```python
from build123d import *

# Parameters (mm, degrees)
F2_W     = 4.6
F2_H     = 45
F3_DEPTH = 12.5
F4_W     = 4.6
F4_H     = 45
F5_DEPTH = 12.5


with BuildPart() as f1:
    # F0 (on Right) → F1 (revolve)
    with BuildSketch(Plane.YZ):
        Polygon((-6, 0), (-6, 50), (-8, 50), (-8, 0.018575), (-3.663243, -12), (-2.5, -12), (-2.5, -9.5), align=None)
    revolve(axis=Axis((0, 0, 4.996806), (0, 0, -1)))

    # F2 (on Front) → F3 (cut, symmetric)
    with BuildSketch(Plane.XZ):
        with Locations((0, 22.5)):
            Rectangle(F2_W, F2_H)
    extrude(amount=F3_DEPTH, both=True, mode=Mode.SUBTRACT)

    # F4 (on Right) → F5 (cut, symmetric)
    with BuildSketch(Plane.YZ):
        with Locations((0, 22.5)):
            Rectangle(F4_W, F4_H)
    extrude(amount=F5_DEPTH, both=True, mode=Mode.SUBTRACT)


solid = f1.part
```
Check sheet for the modelled part. Datum: model origin and axes. Units: mm. A direction names the side the tool comes from. Give positions to 0.01 mm unless a question says otherwise; leave off trailing zeros. Loops run counter-clockwise (first coordinate to the right, second up) from the corner with the lowest first, then second, coordinate; pieces in that order, holes last. Notation, with made-up numbers: M 77,45.25 L 136,45.25 A31 cw 136,75.25 Z; hole C 8.5,-11 d3. An arc over 180 degrees is marked long. Answer in a Markdown table with one row per item.
1) Thickness scan on line 1 (X direction, y = -3.5, z = 37.5); line 2 (X direction, y = 0, z = -10.85); line 3 (Y direction, x = -6, z = 39). Record the ranges inside material, lowest first.
Solutions:
| item | result |
|---|---|
| line 1 | x = -7.19 to -4.87, 4.87 to 7.19 |
| line 2 | x = -4.08 to -2.5, 2.5 to 4.08 |
| line 3 | y = -5.29 to -2.3, 2.3 to 5.29 |
2) Cross-section at A-A (z = 12). Enter the section's corners in (x, y), plus the area to 3 significant figures.
Solutions:
| item | result |
|---|---|
| outline | M -7.66,-2.3 A8 ccw -2.3,-7.66 L -2.3,-5.54 A6 cw -5.54,-2.3 Z; M -7.66,2.3 L -5.54,2.3 A6 cw -2.3,5.54 L -2.3,7.66 A8 ccw Z; M 2.3,-7.66 A8 ccw 7.66,-2.3 L 5.54,-2.3 A6 cw 2.3,-5.54 Z; M 2.3,5.54 A6 cw 5.54,2.3 L 7.66,2.3 A8 ccw 2.3,7.66 Z |
| area | 50.5 mm^2 |
3) Cross-section at B-B (x = 0). Enter the section's corners in (y, z).
Solutions:
| item | result |
|---|---|
| outline | M -8,45 L -6,45 L -6,50 L -8,50 Z; M -7.99,0 L -3.66,-12 L -2.5,-12 L -2.5,-9.5 L -6,0 Z; M 2.5,-12 L 3.66,-12 L 7.99,0 L 6,0 L 2.5,-9.5 Z; M 6,45 L 8,45 L 8,50 L 6,50 Z |
4) Depth check by flat-ended pin: pin 1 (1.1 mm diameter, centred on y = 6.5, z = 13, fed in from -X); pin 2 (4 mm diameter, centred on y = -1.5, z = -1.5, fed in from +X); pin 3 (7 mm diameter, centred on x = 0, y = 0, fed in from -Z); pin 4 (0.6 mm diameter, centred on x = -6.5, z = 22, fed in from +Y). Enter the tip coordinate at first touch or a pass-through.
Solutions:
| item | result |
|---|---|
| pin 1 | stops at x = -5.35 |
| pin 2 | stops at x = 7.99 |
| pin 3 | stops at z = -12 |
| pin 4 | stops at y = 5.06 |
5) Tool access check on faces 1 (the face through (-7, 0, 45)), 2 (the face through (-2.3, 7, 22)), 3 (the face through (3.65, 4.76, 25.35)), 4 (the face through (3.06, -7.39, 24.66)). Record the directions out of +Z, -Z, +X, -X, +Y, -Y that give a thin tool (end or side, any length) a straight path to the whole face; none if there is none.
Solutions:
| item | result |
|---|---|
| face 1 | +X, -X |
| face 2 | +Y, -Y |
| face 3 | +Z |
| face 4 | +Z, -Z |
6) Mould release check, pull along Z, two halves, no side actions. Record for faces 5 (the face through (2, -2, -12)), 6 (the face through (2.364, 3.083, -5.739)), 7 (the face through (-7, -2.3, 22)), 8 (the face through (7, 0, 45)): released by +Z, released by -Z, zero draft, split by the parting line, or undercut.
Solutions:
| item | result |
|---|---|
| face 5 | released by -Z |
| face 6 | released by +Z |
| face 7 | undercut |
| face 8 | undercut |
7) Cross-section at D-D (z = -2). Enter the section's corners in (x, y).
Solutions:
| item | result |
|---|---|
| outline | C 0,0 d14.54; hole C 0,0 d10.53 |
